```python
from build123d import *

# Parameters (mm, degrees)
SKETCH1_W           = 57.15
SKETCH1_H           = 57.15
SKETCH1_R           = 12.7
BOSS_EXTRUDE1_DEPTH = 6.35
SKETCH2_R           = 1.5875
CUT_EXTRUDE1_DEPTH  = 12.7


with BuildPart() as part:
    # Sketch1 → Boss-Extrude1 (new body)
    with BuildSketch(Plane(origin=(0, 0, 0), x_dir=(1, 0, 0), z_dir=(0, 1, 0))):
        Rectangle(SKETCH1_W, SKETCH1_H)
        Circle(SKETCH1_R, mode=Mode.SUBTRACT)
    extrude(amount=BOSS_EXTRUDE1_DEPTH)

    # Sketch2 → Cut-Extrude1 (cut)
    with BuildSketch(Plane.XY.offset(28.575)):
        with Locations((-19.05, 3.175)):
            Circle(SKETCH2_R)
        with Locations((19.05, 3.175)):
            Circle(SKETCH2_R)
    extrude(amount=-CUT_EXTRUDE1_DEPTH, mode=Mode.SUBTRACT)


solid = part.part
```
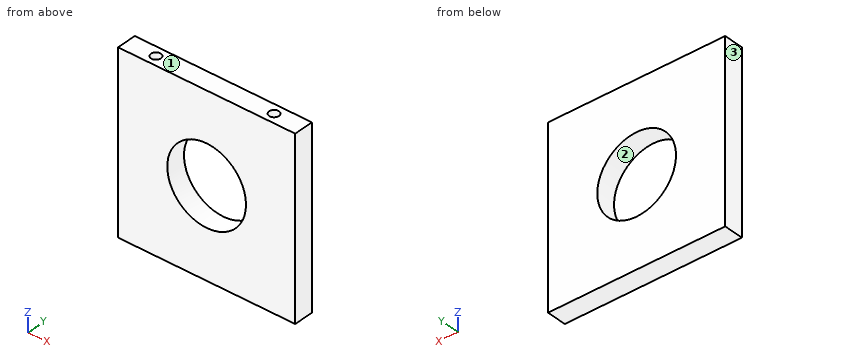
Here's how the part is built. I have some questions about the finished solid (model axes, mm). Face numbers are marked on the shaded views. Give positions to 0.01 mm unless a question says otherwise; leave off trailing zeros. Write each loop counter-clockwise with the first axis right and the second up, starting at its lowest first coordinate (ties: lowest second). Pieces come first, ordered by that corner, then holes. Notation, with made-up numbers: (-24, -36) -> (5, -36) arc R20 cw to (5, -24) -> close; hole circle Ø8 at (18, 60). An arc over 180 degrees is marked (long way). Write each question's results on one line, items separated by ' | '.
Item 1: Suppose I cut it at A-A on x = 0. Write out the boundary of the cut face in (y, z) (3 decimals).
Output:
outline: (0, -28.575) -> (6.35, -28.575) -> (6.35, -12.7) -> (0, -12.7) -> close; (0, 12.7) -> (6.35, 12.7) -> (6.35, 28.575) -> (0, 28.575) -> close
Item 2: Suppose I cut it at B-B on z = 0. Write out the boundary of the cut face in (x, y) (3 decimals), plus the area to 3 significant figures.
Output:
outline: (-28.575, 0) -> (-12.7, 0) -> (-12.7, 6.35) -> (-28.575, 6.35) -> close; (12.7, 0) -> (28.575, 0) -> (28.575, 6.35) -> (12.7, 6.35) -> close | area: 202 mm^2
Item 3: If I drill on L1, parallel to Y at x = -19.05, z = 26.25; L2, parallel to X at y = 4, z = 0 (3 decimals); L3, parallel to Z at x = 0.5, y = 1 (3 decimals), over which ranges is the centre line in solid material (lowest first)?
Output:
L1: y = 0 to 1.59, 4.76 to 6.35 | L2: x = -28.575 to -12.7, 12.7 to 28.575 | L3: z = -28.575 to -12.69, 12.69 to 28.575
Item 4: Suppose I cut it at D-D on z = 19.5. Give the number of separate pieces and of enclosed holes in the cut face, plus the area to 3 significant figures.
Output:
separate pieces: 1 | enclosed holes: 2 | area: 347 mm^2
Item 5: For pin 1 Ø1.5 at (x, z) = (20.5, -7.5) entering from -Y; pin 2 Ø3 at (x, y) = (-19.05, 3.175) entering from +Z (3 decimals), each with a flat end and sliding along its axis, tell me the tip position at first contact or that it passes through.
Output:
pin 1: stops at y = 0 | pin 2: stops at z = 15.875
Item 6: We'd pull the mould along Z, two halves only. Please class the marked faces 1, 2 and 3: pulls with the +Z half, pulls with the -Z half, needs draft (parallel to the pull), parting line crosses it, or undercut.
Output:
face 1: pulls with the +Z half | face 2: undercut | face 3: needs draft
